Source: CAD feature listing. Evaluate the final solid. Frame: model axes, mm. A direction names the side the tool comes from. Coordinates: 2 decimals unless noted, no trailing zeros. Loops run counter-clockwise (first coordinate to the right, second up) from the corner with the lowest first, then second, coordinate; pieces in that order, holes last.
Item 1: Pull-direction query (X, two-part tool) for faces 4 (the flat face through (35, -35, -12)), 5 (the flat face through (-43, -42, -13)), 6 (the cylindrical face through (37.506, 38.728, -5.916)), 7 (the cylindrical face through (-49.08, 38.61, -11.37)); classes: +X half, -X half, draft (parallel to the pull), parting line (faces both ways), or undercut.
Item 2: Reachability of faces 1 (the cylindrical face through (37, -39, -6)), 2 (the flat face through (43, -42, -97)), 3 (the cylindrical face through (-49.08, -41.56, -101.33)) from +Z, -Z, +X, -X, +Y, -Y: full face, straight path, thin tool, end or side. Return the list, or none.
Item 3: Section query A-A, the plane z = -55. Return the cut outline in (x, y).
Item 4: Section query D-D, the plane y = 28. Return the cut outline in (x, z), then the cut area to 3 significant figures.
Item 5: Pin query (flat end, axial travel): pin 1 Ø1 at (x, y) = (-28, -7.5) entering from +Z; pin 2 Ø6.5 at (x, y) = (-35.36, 35.36) entering from +Z; pin 3 Ø6.5 at (y, z) = (42.43, -97.43) entering from -X. Return the tip coordinate at first contact, or that it passes through.
Item 6: Section query C-C, the plane x = 0. Return the cut outline in (y, z), then the cut area to 3 significant figures.
Item 7: Section query B-B, the plane y = 0. Return the cut outline in (x, z), then the cut area to 3 significant figures.
Item 8: Line query: probe 1 along Y at (x, z) = (46, -64); probe 2 along Z at (x, y) = (-41.5, 1); probe 3 along Z at (x, y) = (53, 0). Output: solid intervals per line, ascending.
```python
from build123d import *

# Parameters (mm, degrees)
F0_W      = 110
F0_H      = 110
F0_R      = 4
F0_R_2    = 40
F0_R_3    = 36.5
F1_DEPTH  = 110
F2_DEPTH  = 2.4
F3_DEPTH  = 36.5
F4_DEPTH  = 12
F5_R      = 41
F6_DEPTH  = 110.001
F5_R_2    = 45
F7_DEPTH  = 2.4
F5_R_3    = 4
F8_DEPTH  = 12
F9_R      = 45
F9_R_2    = 41
F10_DEPTH = 2.4
F9_R_3    = 4
F11_DEPTH = 12


with BuildPart() as f1:
    # F0 (on Top) → F1 (new body)
    with BuildSketch(Plane.XY):
        Rectangle(F0_W, F0_H)
        with Locations((-35.3553390593, -35.3553390593)):
            Circle(F0_R, mode=Mode.SUBTRACT)
        with Locations((35.3553390593, -35.3553390593)):
            Circle(F0_R, mode=Mode.SUBTRACT)
        with Locations((-35.3553390593, 35.3553390593)):
            Circle(F0_R, mode=Mode.SUBTRACT)
        Circle(F0_R_2, mode=Mode.SUBTRACT)
        with Locations((35.3553390593, 35.3553390593)):
            Circle(F0_R, mode=Mode.SUBTRACT)
        Circle(F0_R_2)
        Circle(F0_R_3, mode=Mode.SUBTRACT)
        Circle(F0_R_3)
        with Locations((35.3553390593, -35.3553390593)):
            Circle(F0_R)
        with Locations((-35.3553390593, -35.3553390593)):
            Circle(F0_R)
        with Locations((-35.3553390593, 35.3553390593)):
            Circle(F0_R)
        with Locations((35.3553390593, 35.3553390593)):
            Circle(F0_R)
    extrude(amount=-F1_DEPTH)

    # F0 (on Top) → F2 (cut)
    with BuildSketch(Plane.XY):
        Circle(F0_R_2)
        Circle(F0_R_3, mode=Mode.SUBTRACT)
    extrude(amount=-F2_DEPTH, mode=Mode.SUBTRACT)

    # F0 (on Top) → F3 (cut)
    with BuildSketch(Plane.XY):
        Circle(F0_R_3)
    extrude(amount=-F3_DEPTH, mode=Mode.SUBTRACT)

    # F0 (on Top) → F4 (cut)
    with BuildSketch(Plane.XY):
        with Locations((35.3553390593, 35.3553390593)):
            Circle(F0_R)
        with Locations((-35.3553390593, 35.3553390593)):
            Circle(F0_R)
        with Locations((-35.3553390593, -35.3553390593)):
            Circle(F0_R)
        with Locations((35.3553390593, -35.3553390593)):
            Circle(F0_R)
    extrude(amount=-F4_DEPTH, mode=Mode.SUBTRACT)

    # F5 (on face) → F6 (cut, through all)
    with BuildSketch(Plane.YZ.offset(55)):
        with Locations((0, -55)):
            Circle(F5_R)
    extrude(amount=-F6_DEPTH, mode=Mode.SUBTRACT)

    # F5 (on face) → F7 (cut)
    with BuildSketch(Plane.YZ.offset(55)):
        with Locations((0, -55)):
            Circle(F5_R_2)
        with Locations((0, -55)):
            Circle(F5_R, mode=Mode.SUBTRACT)
    extrude(amount=-F7_DEPTH, mode=Mode.SUBTRACT)

    # F5 (on face) → F8 (cut)
    with BuildSketch(Plane.YZ.offset(55)):
        with Locations((42.4264068712, -12.5735931288)):
            Circle(F5_R_3)
        with Locations((-42.4264068712, -12.5735931288)):
            Circle(F5_R_3)
        with Locations((-42.4264068712, -97.4264068712)):
            Circle(F5_R_3)
        with Locations((42.4264068712, -97.4264068712)):
            Circle(F5_R_3)
    extrude(amount=-F8_DEPTH, mode=Mode.SUBTRACT)

    # F9 (on face) → F10 (cut)
    with BuildSketch(Plane(origin=(-55, 0, 0), x_dir=(0, -1, 0), z_dir=(-1, 0, 0))):
        with Locations((0, -55)):
            Circle(F9_R)
        with Locations((0, -55)):
            Circle(F9_R_2, mode=Mode.SUBTRACT)
    extrude(amount=-F10_DEPTH, mode=Mode.SUBTRACT)

    # F9 (on face) → F11 (cut)
    with BuildSketch(Plane(origin=(-55, 0, 0), x_dir=(0, -1, 0), z_dir=(-1, 0, 0))):
        with Locations((-42.4264068712, -12.5735931288)):
            Circle(F9_R_3)
        with Locations((42.4264068712, -12.5735931288)):
            Circle(F9_R_3)
        with Locations((42.4264068712, -97.4264068712)):
            Circle(F9_R_3)
        with Locations((-42.4264068712, -97.4264068712)):
            Circle(F9_R_3)
    extrude(amount=-F11_DEPTH, mode=Mode.SUBTRACT)


solid = f1.part
```
Verdict:
1. face 4: undercut
1. face 5: -X half
1. face 6: undercut
1. face 7: draft
2. face 1: +Z
2. face 2: +X
2. face 3: -X
3. outline: (-55, -55) - (55, -55) - (55, -45) - (52.6, -45) - (52.6, -41) - (-52.6, -41) - (-52.6, -45) - (-55, -45) - close; (-55, 45) - (-52.6, 45) - (-52.6, 41) - (52.6, 41) - (52.6, 45) - (55, 45) - (55, 55) - (-55, 55) - close
4. outline: (-55, -110) - (55, -110) - (55, -90.23) - (52.6, -90.23) - (52.6, -84.95) - (-52.6, -84.95) - (-52.6, -90.23) - (-55, -90.23) - close; (-55, -19.77) - (-52.6, -19.77) - (-52.6, -25.05) - (-23.41, -25.05) - (-23.41, -2.4) - (-28.57, -2.4) - (-28.57, 0) - (-55, 0) - close; (23.41, -25.05) - (52.6, -25.05) - (52.6, -19.77) - (55, -19.77) - (55, 0) - (28.57, 0) - (28.57, -2.4) - (23.41, -2.4) - close
4. area: 4,260 mm2
5. pin 1: stops at z = -95.21
5. pin 2: stops at z = -12
5. pin 3: stops at x = -43
6. outline: (-55, -110) - (55, -110) - (55, 0) - (40, 0) - (40, -2.4) - (36.5, -2.4) - (36.5, -36.33) arc R41 cw (long way) to (-36.5, -36.33) - (-36.5, -2.4) - (-40, -2.4) - (-40, 0) - (-55, 0) - close
6. area: 5,310 mm2
7. outline: (-55, -110) - (55, -110) - (55, -100) - (52.6, -100) - (52.6, -96) - (-52.6, -96) - (-52.6, -100) - (-55, -100) - close; (-55, -10) - (-52.6, -10) - (-52.6, -14) - (-36.5, -14) - (-36.5, -2.4) - (-40, -2.4) - (-40, 0) - (-55, 0) - close; (36.5, -14) - (52.6, -14) - (52.6, -10) - (55, -10) - (55, 0) - (40, 0) - (40, -2.4) - (36.5, -2.4) - close
7. area: 2,000 mm2
8. probe 1: y = -55 to -40, 40 to 55
8. probe 2: z = -110 to -95.99, -14.01 to 0
8. probe 3: z = -110 to -100, -10 to 0
